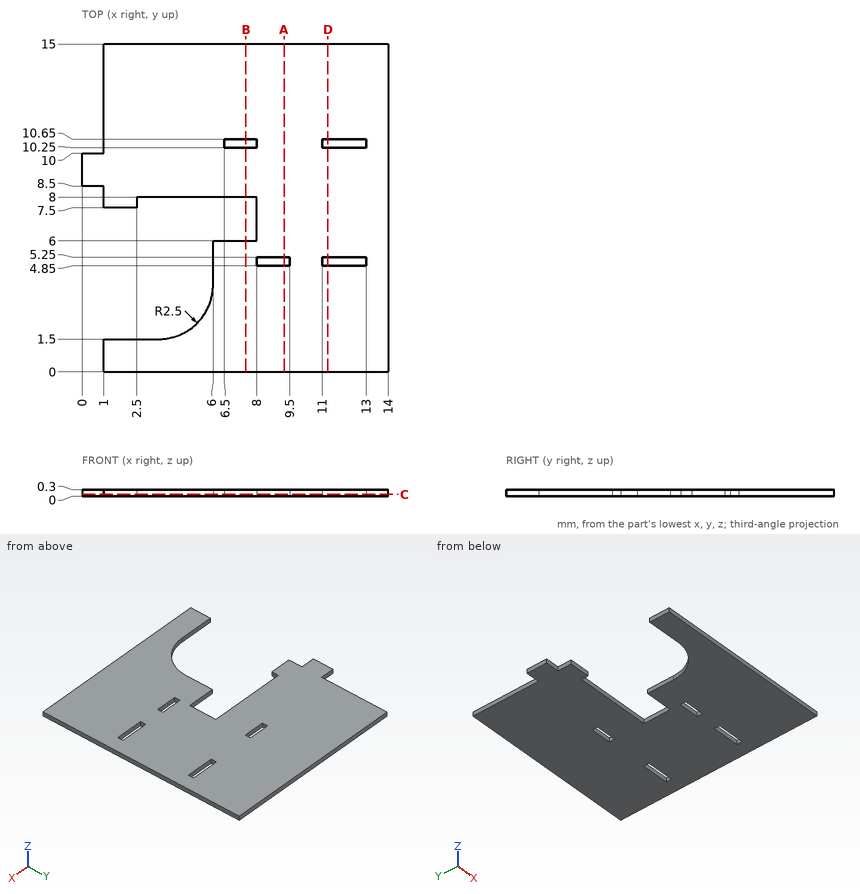
Geometry check sheet. Reference: drawing and pictorial views, mm from the part's lowest x, y, z. Round coordinates to 2 decimals unless told otherwise and drop trailing zeros. Loops run counter-clockwise (first coordinate to the right, second up) from the corner with the lowest first, then second, coordinate; pieces in that order, holes last. Notation, with made-up numbers: M 4,-20 L 26,-20 A19 cw 26,7 Z; hole C 22.25,81.25 d4. An arc over 180 degrees is marked long. Return JSON: item names as keys, results as strings. Group by question number.
(1) Section check B-B, the plane x = 7.5. Enter the section's corners in (y, z), and give its area (3 significant figures).
(2) Section check D-D, the plane x = 11.25. Enter the section's corners in (y, z), and give its area (3 significant figures).
(3) Scan lines: line 1 along Y through (x, z) = (6.75, 0.25); line 2 along X through (y, z) = (10.5, 0.15); line 3 along Y through (x, z) = (11.75, 0.1). Record each from-to range of solid material in increasing order. Write a range as [from, to].
(4) Section check C-C, the plane z = 0.1. Give the number of separate pieces and of enclosed holes in the cut face, and give its area (3 significant figures).
(5) Section check A-A, the plane x = 9.25. Enter the section's corners in (y, z).
Data:
{
 "1": {"outline": "M 0,0 L 6,0 L 6,0.3 L 0,0.3 Z; M 8,0 L 10.25,0 L 10.25,0.3 L 8,0.3 Z; M 10.65,0 L 15,0 L 15,0.3 L 10.65,0.3 Z", "area": "3.78 mm²"},
 "2": {"outline": "M 0,0 L 4.85,0 L 4.85,0.3 L 0,0.3 Z; M 5.25,0 L 10.25,0 L 10.25,0.3 L 5.25,0.3 Z; M 10.65,0 L 15,0 L 15,0.3 L 10.65,0.3 Z", "area": "4.26 mm²"},
 "3": {"line 1": "[0, 6], [8, 10.25], [10.65, 15]", "line 2": "[1, 6.5], [8, 11], [13, 14]", "line 3": "[0, 4.85], [5.25, 10.25], [10.65, 15]"},
 "4": {"separate pieces": "1", "enclosed holes": "4", "area": "159 mm²"},
 "5": {"outline": "M 0,0 L 4.85,0 L 4.85,0.3 L 0,0.3 Z; M 5.25,0 L 15,0 L 15,0.3 L 5.25,0.3 Z"}
}
